Geometry: final body of the model. Coordinates: model frame, mm. A direction names the side the tool comes from. Give positions to 0.01 mm unless a question says otherwise; leave off trailing zeros. Write each loop counter-clockwise with the first axis right and the second up, starting at its lowest first coordinate (ties: lowest second). Pieces come first, ordered by that corner, then holes.
Q1. Reachability of faces 5 (the face through (-160.066, 11, 0)), 6 (the face through (-269.36, 9.71, -2.41)), 7 (the face through (-247, 11.906, 1)), 8 (the face through (-261, 5.556, -8)) from +Z, -Z, +X, -X, +Y, -Y: full face, straight path, thin tool, end or side. Return the list, or none.
Q2. Cut plane B-B on z = -39. Return the cut outline in (x, y), plus the area to 3 significant figures.
Q3. Cut plane A-A on z = 0. Return the cut outline in (x, y) (3 decimals).
Q4. Cut plane C-C on y = 15.5. Return the cut outline in (x, z).
Q5. Pin query (flat end, axial travel): pin 1 (5.5 mm diameter, centred on x = -145.33, z = 41.28, fed in from +Y); pin 2 (3 mm diameter, centred on y = 9.5, z = 23, fed in from -X); pin 3 (11 mm diameter, centred on x = -173.51, z = 39.37, fed in from -Y); pin 4 (8 mm diameter, centred on x = -151.5, y = 13.5, fed in from -Z). Return the tip coordinate at first contact, or that it passes through.
Q6. Line query: L1, parallel to X at y = 2.75, z = -24.13; L2, parallel to X at y = 10.3, z = 0; L3, parallel to X at y = 2.4, z = 0. Output: solid intervals per line, ascending.
Q7. Cut plane D-D on x = -185.5. Return the cut outline in (y, z).
Q8. Draft query along Z for faces 1 (the face through (-151, 13, -31.75)), 2 (the face through (-208, 6.35, -1)), 3 (the face through (-148, 3.175, 0)), 4 (the face through (-208, 3, 50.8)). Return one class per face: pulls with the +Z half, pulls with the -Z half, needs draft (parallel to the pull), parting line crosses it, or undercut.
```python
from build123d import *

# Parameters (mm, degrees)
SKETCH1_W                = 279.4
SKETCH1_H                = 101.6
BOSS_EXTRUDE1_DEPTH      = 6.35
SKETCH2_R                = 13.97
BOSS_EXTRUDE3_DEPTH      = 5.55625
SKETCH9_R                = 11.1125
CUT_EXTRUDE4_DEPTH       = 4.445
CUT_EXTRUDE5_START       = -5.55625
SKETCH10_R               = 11.1125
CUT_EXTRUDE5_DEPTH       = 5.55625
SKETCH11_R               = 7.9375
CUT_EXTRUDE6_DEPTH       = 285.078633923
SKETCH12_R               = 6.35
CUT_EXTRUDE7_DEPTH       = 285.051619429
SKETCH22_W               = 63.5
SKETCH22_H               = 63.5
BOSS_EXTRUDE7_DEPTH      = 12.7
SKETCH25_W               = 50.8
SKETCH25_H               = 50.8
CUT_EXTRUDE11_DEPTH      = 15.875
SKETCH32_R               = 4.7625
CUT_EXTRUDE12_DEPTH      = 6.35
SKETCH38_W               = 46.99
SKETCH38_H               = 18.470251096
CUT_EXTRUDE13_DEPTH      = 6.35
SKETCH60_R               = 4.7625
CUT_EXTRUDE23_DEPTH      = 6.35
SKETCH64_R               = 4.7625
CUT_EXTRUDE24_DEPTH      = 285.264471927
SKETCH69_W               = 33.02
SKETCH69_H               = 6.35
BOSS_EXTRUDE10_DEPTH     = 19.05
SKETCH70_R               = 4.7625
SKETCH70_R_2             = 2.54
CUT_EXTRUDE26_DEPTH      = 6.35
SKETCH76_R               = 4.7625
CUT_EXTRUDE29_DEPTH      = 6.35
SKETCH77_W               = 46.99
SKETCH77_H               = 16.7871648
CUT_EXTRUDE30_DEPTH      = 6.35
SKETCH78_W               = 49.276
SKETCH78_H               = 66.342584104
CUT_EXTRUDE32_DEPTH      = 1.524
SKETCH79_R               = 4.7625
CUT_EXTRUDE33_DEPTH      = 4.826
CUT_EXTRUDE34_DEPTH      = 289.436124861
CUT_EXTRUDE34_DEPTH_BACK = 289.436124861


with BuildPart() as part:
    # Sketch1 → Boss-Extrude1 (new body)
    with BuildSketch(Plane(origin=(0, 0, 0), x_dir=(1, 0, 0), z_dir=(0, 1, 0))):
        with Locations((-139.7, 0)):
            Rectangle(SKETCH1_W, SKETCH1_H)
    extrude(amount=BOSS_EXTRUDE1_DEPTH)

    # Sketch2 → Boss-Extrude3 (add)
    with BuildSketch(Plane(origin=(0, 6.35, 0), x_dir=(1, 0, 0), z_dir=(0, 1, 0))):
        with Locations(Location((-258.510557857, 0, 0), (0, 0, 90))):
            Circle(SKETCH2_R)
    extrude(amount=BOSS_EXTRUDE3_DEPTH)

    # Sketch9 → Cut-Extrude4 (cut)
    with BuildSketch(Plane(origin=(0, 11.90625, 0), x_dir=(1, 0, 0), z_dir=(0, 1, 0))):
        with Locations(Location((-258.510557857, 0, 0), (0, 0, 270))):
            Circle(SKETCH9_R)
    extrude(amount=-CUT_EXTRUDE4_DEPTH, mode=Mode.SUBTRACT)

    # Sketch10 → Cut-Extrude5 (cut)
    with BuildSketch(Plane(origin=(0, 0, 0), x_dir=(-1, 0, 0), z_dir=(0, -1, 0)).offset(CUT_EXTRUDE5_START)):
        with Locations(Location((258.510557857, 0, 0), (0, 0, 270))):
            Circle(SKETCH10_R)
    extrude(amount=CUT_EXTRUDE5_DEPTH, mode=Mode.SUBTRACT)

    # Sketch11 → Cut-Extrude6 (cut, through all)
    with BuildSketch(Plane(origin=(0, 7.46125, 0), x_dir=(1, 0, 0), z_dir=(0, 1, 0))):
        with Locations(Location((-258.510557857, 0, 0), (0, 0, 270))):
            Circle(SKETCH11_R)
    extrude(amount=-CUT_EXTRUDE6_DEPTH, mode=Mode.SUBTRACT)

    # Sketch12 → Cut-Extrude7 (cut, through all)
    with BuildSketch(Plane(origin=(0, 6.35, 0), x_dir=(1, 0, 0), z_dir=(0, 1, 0))):
        with Locations(Location((-134.666203771, 0, 0), (0, 0, 270))):
            Circle(SKETCH12_R)
    extrude(amount=-CUT_EXTRUDE7_DEPTH, mode=Mode.SUBTRACT)

    # Sketch22 → Boss-Extrude7 (add)
    with BuildSketch(Plane(origin=(0, 6.35, 0), x_dir=(1, 0, 0), z_dir=(0, 1, 0))):
        with Locations((-134.666203771, 0)):
            Rectangle(SKETCH22_W, SKETCH22_H)
    extrude(amount=BOSS_EXTRUDE7_DEPTH)

    # Sketch25 → Cut-Extrude11 (cut)
    with BuildSketch(Plane(origin=(0, 19.05, 0), x_dir=(1, 0, 0), z_dir=(0, 1, 0))):
        with Locations((-134.666203771, 0)):
            Rectangle(SKETCH25_W, SKETCH25_H)
    extrude(amount=-CUT_EXTRUDE11_DEPTH, mode=Mode.SUBTRACT)

    # Sketch32 → Cut-Extrude12 (cut)
    with BuildSketch(Plane(origin=(0, 6.35, 0), x_dir=(1, 0, 0), z_dir=(0, 1, 0))):
        with Locations(Location((-67.44195898, -40.64, 0), (0, 0, 270))):
            Circle(SKETCH32_R)
        with Locations(Location((-81.41195898, -40.64, 0), (0, 0, 270))):
            Circle(SKETCH32_R)
        with Locations(Location((-67.44195898, 40.64, 0), (0, 0, 270))):
            Circle(SKETCH32_R)
        with Locations(Location((-81.41195898, 40.64, 0), (0, 0, 270))):
            Circle(SKETCH32_R)
    extrude(amount=-CUT_EXTRUDE12_DEPTH, mode=Mode.SUBTRACT)

    # Sketch38 → Cut-Extrude13 (cut)
    with BuildSketch(Plane(origin=(0, 6.35, 0), x_dir=(1, 0, 0), z_dir=(0, 1, 0))):
        with Locations((-23.495, -24.777709652)):
            Rectangle(SKETCH38_W, SKETCH38_H)
    extrude(amount=-CUT_EXTRUDE13_DEPTH, mode=Mode.SUBTRACT)

    # Sketch60 → Cut-Extrude23 (cut)
    with BuildSketch(Plane(origin=(0, 6.35, 0), x_dir=(1, 0, 0), z_dir=(0, 1, 0))):
        with Locations(Location((-231.7492444, 41.324145444, 0), (0, 0, 270))):
            Circle(SKETCH60_R)
        with Locations(Location((-231.7492444, -39.369341378, 0), (0, 0, 270))):
            Circle(SKETCH60_R)
        with Locations(Location((-173.509244294, -39.369341378, 0), (0, 0, 270))):
            Circle(SKETCH60_R)
        with Locations(Location((-173.509244294, 41.324145444, 0), (0, 0, 270))):
            Circle(SKETCH60_R)
    extrude(amount=-CUT_EXTRUDE23_DEPTH, mode=Mode.SUBTRACT)

    # Sketch64 → Cut-Extrude24 (cut, through all)
    with BuildSketch(Plane(origin=(0, 6.35, 0), x_dir=(1, 0, 0), z_dir=(0, 1, 0))):
        with Locations(Location((-145.334203771, -41.275, 0), (0, 0, 270))):
            Circle(SKETCH64_R)
        with Locations(Location((-123.998203771, -41.275, 0), (0, 0, 270))):
            Circle(SKETCH64_R)
    cut_extrude24 = extrude(amount=-CUT_EXTRUDE24_DEPTH, mode=Mode.SUBTRACT)

    # Mirror1: Cut-Extrude24 across plane
    add(cut_extrude24.mirror(Plane.XY), mode=Mode.SUBTRACT)

    # Sketch69 → Boss-Extrude10 (add)
    with BuildSketch(Plane.XY.offset(50.8)):
        with Locations((-70.465355554, 3.175)):
            Rectangle(SKETCH69_W, SKETCH69_H)
    boss_extrude10 = extrude(amount=BOSS_EXTRUDE10_DEPTH)

    # Sketch70 → Cut-Extrude26 (cut)
    with BuildSketch(Plane(origin=(0, 6.35, 0), x_dir=(1, 0, 0), z_dir=(0, 1, 0))):
        with Locations(Location((-76.815355554, -60.325, 0), (0, 0, 270))):
            Circle(SKETCH70_R)
        with Locations(Location((-64.115355554, -60.325, 0), (0, 0, 270))):
            Circle(SKETCH70_R_2)
    cut_extrude26 = extrude(amount=-CUT_EXTRUDE26_DEPTH, mode=Mode.SUBTRACT)

    # Mirror2: Boss-Extrude10, Cut-Extrude26 across plane
    add(boss_extrude10.mirror(Plane.XY))
    add(cut_extrude26.mirror(Plane.XY), mode=Mode.SUBTRACT)

    # Sketch76 → Cut-Extrude29 (cut)
    with BuildSketch(Plane(origin=(0, 6.35, 0), x_dir=(1, 0, 0), z_dir=(0, 1, 0))):
        with Locations(Location((-264.668, 24.13, 0), (0, 0, 270))):
            Circle(SKETCH76_R)
        with Locations(Location((-252.222, 24.13, 0), (0, 0, 270))):
            Circle(SKETCH76_R)
    extrude(amount=-CUT_EXTRUDE29_DEPTH, mode=Mode.SUBTRACT)

    # Sketch77 → Cut-Extrude30 (cut)
    with BuildSketch(Plane(origin=(0, 6.35, 0), x_dir=(1, 0, 0), z_dir=(0, 1, 0))):
        with Locations((-23.495, -42.4064176)):
            Rectangle(SKETCH77_W, SKETCH77_H)
    extrude(amount=-CUT_EXTRUDE30_DEPTH, mode=Mode.SUBTRACT)

    # Sketch78 → Cut-Extrude32 (cut)
    with BuildSketch(Plane(origin=(0, 6.35, 0), x_dir=(1, 0, 0), z_dir=(0, 1, 0))):
        with Locations((-24.638, 17.628707948)):
            Rectangle(SKETCH78_W, SKETCH78_H)
    extrude(amount=-CUT_EXTRUDE32_DEPTH, mode=Mode.SUBTRACT)

    # Sketch79 → Cut-Extrude33 (cut)
    with BuildSketch(Plane(origin=(0, 4.826, 0), x_dir=(1, 0, 0), z_dir=(0, 1, 0))):
        with Locations(Location((-23.876, 15.191415896, 0), (0, 0, 270))):
            Circle(SKETCH79_R)
    extrude(amount=-CUT_EXTRUDE33_DEPTH, mode=Mode.SUBTRACT)

    # Sketch80 → Cut-Extrude34 (cut, two sides: drawn at the far end of the back side and taken through both)
    with BuildSketch(Plane(origin=(0, 3.175, 0), x_dir=(1, 0, 0), z_dir=(0, 1, 0)).offset(-CUT_EXTRUDE34_DEPTH_BACK)):
        Polygon((-134.666203771, 437.651664562), (-134.666203771, 50.8), (-134.666203771, 0), (-134.666203771, -50.8), (-134.666203771, -437.651664562), (639.037125352, -437.651664562), (639.037125352, 437.651664562), align=None)
    extrude(amount=CUT_EXTRUDE34_DEPTH + CUT_EXTRUDE34_DEPTH_BACK, mode=Mode.SUBTRACT)


solid = part.part
```
Data:
1. face 5: +X, +Y
1. face 6: +Y
1. face 7: +Z, -Z, -X, +Y
1. face 8: -Y
2. outline: (-279.4, 0) - (-235.91, 0) - (-235.91, 6.35) - (-279.4, 6.35) - close; (-227.59, 0) - (-177.67, 0) - (-177.67, 6.35) - (-227.59, 6.35) - close; (-169.35, 0) - (-149.52, 0) - (-149.52, 6.35) - (-169.35, 6.35) - close; (-141.15, 0) - (-134.67, 0) - (-134.67, 6.35) - (-141.15, 6.35) - close
2. area: 760 mm2
3. outline: (-279.4, 0) - (-269.623, 0) - (-269.623, 5.556) - (-266.448, 5.556) - (-266.448, 7.461) - (-269.623, 7.461) - (-269.623, 11.906) - (-272.481, 11.906) - (-272.481, 6.35) - (-279.4, 6.35) - close; (-250.573, 5.556) - (-247.398, 5.556) - (-247.398, 0) - (-141.016, 0) - (-141.016, 3.175) - (-160.066, 3.175) - (-160.066, 19.05) - (-166.416, 19.05) - (-166.416, 6.35) - (-244.541, 6.35) - (-244.541, 11.906) - (-247.398, 11.906) - (-247.398, 7.461) - (-250.573, 7.461) - close
4. outline: (-166.42, -31.75) - (-134.67, -31.75) - (-134.67, -25.4) - (-160.07, -25.4) - (-160.07, 25.4) - (-134.67, 25.4) - (-134.67, 31.75) - (-166.42, 31.75) - close
5. pin 1: passes through
5. pin 2: stops at x = -166.42
5. pin 3: stops at y = 0
5. pin 4: stops at z = -31.75
6. L1: x = -279.4 to -269.43, -259.91 to -256.98, -247.46 to -134.67
6. L2: x = -272.48 to -269.62, -247.4 to -244.54, -166.42 to -160.07
6. L3: x = -279.4 to -269.62, -247.4 to -141.02
7. outline: (0, -50.8) - (6.35, -50.8) - (6.35, 50.8) - (0, 50.8) - close
8. face 1: pulls with the -Z half
8. face 2: needs draft
8. face 3: undercut
8. face 4: pulls with the +Z half
